Here's how the part is built. I have some questions about the finished solid (model axes, mm). A direction names the side the tool comes from. Coordinates: 2 decimals unless noted, no trailing zeros. Write each loop counter-clockwise with the first axis right and the second up, starting at its lowest first coordinate (ties: lowest second). Pieces come first, ordered by that corner, then holes. Notation, with made-up numbers: M 74.5,-34.5 L 130.5,-34.5 A22 ccw 130.5,-5.5 Z; hole C -31.5,13.5 d4. An arc over 180 degrees is marked long. Use one line per item in the form item = value. Start each with the question number.
1. I want a section at A-A, the plane x = 12.5. List the corners of the cut face in (y, z) for me.
2. Please list where these lines run through material, in increasing order: line 1 along Z through (x, y) = (21.5, 28.5); line 2 along Y through (x, z) = (-11, 9). Write a range as [from, to].
3. I'm going to push a flat-ended pin straight in: pin 1 Ø4 at (x, z) = (-27, -8) entering from +Y. Where does the tip first touch, or does it pass through?
4. On a 3-axis mill with a long thin cutter (end or side, diameter ignored), from which of +Z, -Z, +X, -X, +Y, -Y can I reach the whole of each face in a straight line? I mean faces 4 (the face through (-1, 20, -50)), 5 (the face through (40, 25, 0)). Say none if no direction works.
5. I want a section at C-C, the plane z = -3. List the corners of the cut face in (x, y) for me.
6. I want a section at B-B, the plane y = 29.5. List the corners of the cut face in (x, z) for me.
7. Thinking about a two-plate mould opening in Z: for faces 1 (the face through (36.99, 24.79, 37.15)), 2 (the face through (-0.462, -1.35, -42.575)), 3 (the face through (0, 0, -48)), which applies, released by +Z, released by -Z, zero draft, split by the parting line, or undercut?
from build123d import *

# Parameters (mm, degrees)
SKETCH1_W           = 100
SKETCH1_H           = 100
BOSS_EXTRUDE1_DEPTH = 40
SKETCH2_W           = 80
SKETCH2_H           = 80
CUT_EXTRUDE1_DEPTH  = 30
SKETCH3_W           = 80
SKETCH3_H           = 80
BOSS_EXTRUDE2_DEPTH = 5
FILLET2_R           = 10
FILLET4_R           = 7
FILLET5_R           = 7


with BuildPart() as part:
    # Sketch1 → Boss-Extrude1 (new body)
    with BuildSketch(Plane(origin=(0, 0, 0), x_dir=(1, 0, 0), z_dir=(0, 1, 0))):
        Rectangle(SKETCH1_W, SKETCH1_H)
    extrude(amount=BOSS_EXTRUDE1_DEPTH)

    # Sketch2 → Cut-Extrude1 (cut)
    with BuildSketch(Plane(origin=(0, 40, 0), x_dir=(1, 0, 0), z_dir=(0, 1, 0))):
        Rectangle(SKETCH2_W, SKETCH2_H)
    extrude(amount=-CUT_EXTRUDE1_DEPTH, mode=Mode.SUBTRACT)

    # Sketch3 → Boss-Extrude2 (add)
    with BuildSketch(Plane.XZ):
        Rectangle(SKETCH3_W, SKETCH3_H)
    extrude(amount=BOSS_EXTRUDE2_DEPTH)

    # Fillet2
    fillet2_edges = [part.edges().sort_by_distance(p)[0] for p in [
        (-40, 25, 40),
        (-40, 25, -40),
        (40, 25, -40),
        (40, 25, 40),
        (-50, 20, -50),
        (50, 20, -50),
        (50, 20, 50),
        (-50, 20, 50),
    ]]
    fillet(fillet2_edges, radius=FILLET2_R)

    # Fillet4
    fillet4_edges = [part.edges().sort_by_distance(p)[0] for p in [
        (-40, -2.5, 40),
        (-40, -2.5, -40),
        (40, -2.5, -40),
        (40, -2.5, 40),
    ]]
    fillet(fillet4_edges, radius=FILLET4_R)

    # Fillet5
    # the kernel refuses this fillet: 7 mm, written as the material it adds along each edge
    with BuildSketch(Plane(origin=(-33, 0, 33), x_dir=(-1, 0, 0), z_dir=(0, 0, -1))) as fillet5_piece_1:
        with BuildLine():
            CenterArc((13.708203932, -7), FILLET5_R, 90, 73.398450401)
            Line((7, -5), (6.865835921, -4.96))
            ThreePointArc((6.865835921, -4.96), (6.86, -2.5), (6.86, 0))
            Line((6.86, 0), (7, 0.14))
            Line((7, 0.14), (13.708203932, 0.14))
            Line((13.708203932, 0.14), (13.708203932, 0))
        make_face()
    revolve(axis=Axis((-33, 0, 33), (0, 1, 0)), revolution_arc=90)
    with BuildSketch(Plane(origin=(33, 0, 40), x_dir=(0, 0, 1), z_dir=(-1, 0, 0)), Plane(origin=(40, 0, -33), x_dir=(1, 0, 0), z_dir=(0, 0, 1)), Plane(origin=(-33, 0, -40), x_dir=(0, 0, -1), z_dir=(1, 0, 0)), Plane(origin=(-40, 0, 33), x_dir=(-1, 0, 0), z_dir=(0, 0, -1))) as fillet5_piece_2:
        with BuildLine():
            CenterArc((6.708203932, -7), FILLET5_R, 90, 73.398450401)
            Line((0, -5), (-0.134164079, -4.96))
            ThreePointArc((-0.134164079, -4.96), (-0.14, -2.5), (-0.14, 0))
            Line((-0.14, 0), (0, 0.14))
            Line((0, 0.14), (6.708203932, 0.14))
            Line((6.708203932, 0.14), (6.708203932, 0))
        make_face()
    extrude(amount=66)
    with BuildSketch(Plane(origin=(33, 0, 33), x_dir=(1, 0, 0), z_dir=(0, 0, -1))) as fillet5_piece_3:
        with BuildLine():
            CenterArc((13.708203932, 7), FILLET5_R, 196.601549599, 73.398450401)
            Line((7, 5), (6.865835921, 4.96))
            ThreePointArc((6.865835921, 4.96), (6.86, 2.5), (6.86, 0))
            Line((6.86, 0), (7, -0.14))
            Line((7, -0.14), (13.708203932, -0.14))
            Line((13.708203932, -0.14), (13.708203932, 0))
        make_face()
    revolve(axis=Axis((33, 0, 33), (0, -1, 0)), revolution_arc=90)
    with BuildSketch(Plane(origin=(33, 0, -33), x_dir=(1, 0, 0), z_dir=(0, 0, 1))) as fillet5_piece_4:
        with BuildLine():
            CenterArc((13.708203932, -7), FILLET5_R, 90, 73.398450401)
            Line((7, -5), (6.865835921, -4.96))
            ThreePointArc((6.865835921, -4.96), (6.86, -2.5), (6.86, 0))
            Line((6.86, 0), (7, 0.14))
            Line((7, 0.14), (13.708203932, 0.14))
            Line((13.708203932, 0.14), (13.708203932, 0))
        make_face()
    revolve(axis=Axis((33, 0, -33), (0, 1, 0)), revolution_arc=90)
    with BuildSketch(Plane(origin=(-33, 0, -33), x_dir=(0, 0, -1), z_dir=(1, 0, 0))) as fillet5_piece_5:
        with BuildLine():
            CenterArc((13.708203932, -7), FILLET5_R, 90, 73.398450401)
            Line((7, -5), (6.865835921, -4.96))
            ThreePointArc((6.865835921, -4.96), (6.86, -2.5), (6.86, 0))
            Line((6.86, 0), (7, 0.14))
            Line((7, 0.14), (13.708203932, 0.14))
            Line((13.708203932, 0.14), (13.708203932, 0))
        make_face()
    revolve(axis=Axis((-33, 0, -33), (0, 1, 0)), revolution_arc=90)


solid = part.part
Answer list:
q1.outline = M -5,-40 A7 cw 0,-46.71 L 0,-50 L 40,-50 L 40,-40 L 10,-40 L 10,40 L 40,40 L 40,50 L 0,50 L 0,46.71 A7 cw -5,40 Z
q2.line_1 = [-50, -40], [40, 50]
q2.line_2 = [-5, 10]
q3.pin_1 = 10
q4.face_4 = -Z, +X, -X, +Y, -Y
q4.face_5 = +Y
q5.outline = M -50,0 L -46.71,0 A7 cw -40,-5 L 40,-5 A7 cw 46.71,0 L 50,0 L 50,40 L 40,40 L 40,10 L -40,10 L -40,40 L -50,40 Z
q6.outline = M -50,-40 A10 ccw -40,-50 L 40,-50 A10 ccw 50,-40 L 50,40 A10 ccw 40,50 L -40,50 A10 ccw -50,40 Z; hole M -40,-30 A10 ccw -30,-40 L 30,-40 A10 ccw 40,-30 L 40,30 A10 ccw 30,40 L -30,40 A10 ccw -40,30 Z
q7.face_1 = undercut
q7.face_2 = released by -Z
q7.face_3 = zero draft
